from build123d import *

# Parameters (mm, degrees)
SKETCH1_W           = 2
SKETCH1_H           = 2
SKETCH1_W_2         = 1.6
SKETCH1_H_2         = 1.6
BOSS_EXTRUDE1_DEPTH = 109
SKETCH2_W           = 2
SKETCH2_H           = 2
SKETCH2_W_2         = 1.6
SKETCH2_H_2         = 1.6
BOSS_EXTRUDE2_DEPTH = 34
SKETCH3_W           = 2
SKETCH3_H           = 2
SKETCH3_W_2         = 1.6
SKETCH3_H_2         = 1.6
BOSS_EXTRUDE3_DEPTH = 6
SKETCH7_W           = 2
SKETCH7_H           = 2
SKETCH7_W_2         = 1.54
SKETCH7_H_2         = 1.54
BOSS_EXTRUDE4_DEPTH = 36
BOSS_EXTRUDE5_REACH = 28
SKETCH8_W           = 2
SKETCH8_H           = 2
SKETCH8_W_2         = 1.6
SKETCH8_H_2         = 1.6
SCALE2_SCALE        = 10
BOSS_EXTRUDE6_REACH = 1412
SKETCH9_W           = 20
SKETCH9_H           = 20
SKETCH9_W_2         = 16
SKETCH9_H_2         = 16


with BuildPart() as part:
    # Sketch1 → Boss-Extrude1 (new body)
    with BuildSketch(Plane(origin=(0, 0, 0), x_dir=(1, 0, 0), z_dir=(0, 1, 0))):
        Rectangle(SKETCH1_W, SKETCH1_H)
        Rectangle(SKETCH1_W_2, SKETCH1_H_2, mode=Mode.SUBTRACT)
    boss_extrude1 = extrude(amount=BOSS_EXTRUDE1_DEPTH)

    # Sketch2 → Boss-Extrude2 (add)
    with BuildSketch(Plane.XY.offset(1)):
        with Locations((0, 108)):
            Rectangle(SKETCH2_W, SKETCH2_H)
        with Locations((0, 108)):
            Rectangle(SKETCH2_W_2, SKETCH2_H_2, mode=Mode.SUBTRACT)
    extrude(amount=BOSS_EXTRUDE2_DEPTH)

    # Mirror1: Boss-Extrude1 across plane
    add(boss_extrude1.mirror(Plane.XY.offset(17)))

    # Sketch3 → Boss-Extrude3 (add)
    with BuildSketch(Plane.XY.offset(1)):
        with Locations((0, 1)):
            Rectangle(SKETCH3_W, SKETCH3_H)
        with Locations((0, 1)):
            Rectangle(SKETCH3_W_2, SKETCH3_H_2, mode=Mode.SUBTRACT)
    boss_extrude3 = extrude(amount=BOSS_EXTRUDE3_DEPTH)

    # Sketch7 → Boss-Extrude4 (add)
    with BuildSketch(Plane(origin=(0, 2, 0), x_dir=(1, 0, 0), z_dir=(0, 1, 0))):
        with Locations((0, -8)):
            Rectangle(SKETCH7_W, SKETCH7_H)
        with Locations((0, -8)):
            Rectangle(SKETCH7_W_2, SKETCH7_H_2, mode=Mode.SUBTRACT)
    boss_extrude4 = extrude(amount=-BOSS_EXTRUDE4_DEPTH)

    # Mirror2: Boss-Extrude3, Boss-Extrude4 across plane
    add(boss_extrude3.mirror(Plane.XY.offset(17)))
    add(boss_extrude4.mirror(Plane.XY.offset(17)))

    # Sketch8 → Boss-Extrude5 (add, up to next)
    with BuildSketch(Plane(origin=(0, 0, 25), x_dir=(-1, 0, 0), z_dir=(0, 0, -1)), mode=Mode.PRIVATE) as boss_extrude5_sk1:
        with Locations((0, -33)):
            Rectangle(SKETCH8_W, SKETCH8_H)
        with Locations((0, -33)):
            Rectangle(SKETCH8_W_2, SKETCH8_H_2, mode=Mode.SUBTRACT)
    boss_extrude5_tool1 = extrude(boss_extrude5_sk1.sketch, amount=BOSS_EXTRUDE5_REACH, mode=Mode.PRIVATE) - part.part
    add(boss_extrude5_tool1.solids().sort_by_distance((0, -32.028284, 25))[0])


with BuildPart() as part_1:
    # Scale2: scaled about (0, 0, 0)
    add(part.part.scale(SCALE2_SCALE))

    # Sketch9 → Boss-Extrude6 (add, up to next)
    with BuildSketch(Plane.XZ.offset(-1070), mode=Mode.PRIVATE) as boss_extrude6_sk1:
        with Locations((0, 169.738105544)):
            Rectangle(SKETCH9_W, SKETCH9_H)
        with Locations((0, 169.738105544)):
            Rectangle(SKETCH9_W_2, SKETCH9_H_2, mode=Mode.SUBTRACT)
    boss_extrude6_tool1 = extrude(boss_extrude6_sk1.sketch, amount=BOSS_EXTRUDE6_REACH, mode=Mode.PRIVATE) - part_1.part
    add(boss_extrude6_tool1.solids().sort_by_distance((0, 1070, 179.455263))[0])


solid = part_1.part
The listing builds one solid part. Answer for the finished solid, in the listing's coordinates (mm). Round coordinates to 2 decimals unless told otherwise and drop trailing zeros. Write each loop counter-clockwise with the first axis right and the second up, starting at its lowest first coordinate (ties: lowest second). Pieces come first, ordered by that corner, then holes. Notation, with made-up numbers: M -8,36.5 L 8,36.5 A23 cw 8,54.5 Z; hole C -8,-25 d2. An arc over 180 degrees is marked long. Write each question's results on one line, items separated by ' | '. Start each with the question number.
Item 1: Given pin 1 Ø10 at (x, y) = (-3, -161.5) entering from -Z, flat-ended and moving along its own axis, determine where the tip first touches the part or whether it passes through.
Item 2: Find section A-A on y = 65.5. Write down the section's boundary in (x, z).
Item 3: Find section B-B on z = 120. Write down the section's boundary in (x, y), and give its area (3 significant figures).
Item 4: Straight lines are drawn through the part: probe 1 along Y at (x, z) = (6.5, 213); probe 2 along Y at (x, z) = (-7.25, 322); probe 3 along Z at (x, y) = (1.5, 482). For each, find the intervals that lie inside material, in ascending order.
Item 5: Find section C-C on y = -82. Write down the section's boundary in (x, z).
Answer block:
1) pin 1: stops at z = 70
2) outline: M -10,-10 L 10,-10 L 10,10 L -10,10 Z; M -10,159.74 L 10,159.74 L 10,179.74 L -10,179.74 Z; M -10,330 L 10,330 L 10,350 L -10,350 Z; hole M -8,-8 L 8,-8 L 8,8 L -8,8 Z; hole M -8,161.74 L 8,161.74 L 8,177.74 L -8,177.74 Z; hole M -8,332 L 8,332 L 8,348 L -8,348 Z
3) outline: M -10,-340 L 10,-340 L 10,-320 L -10,-320 Z; M -10,1070 L 10,1070 L 10,1090 L -10,1090 Z; hole M -8,-338 L 8,-338 L 8,-322 L -8,-322 Z; hole M -8,1072 L 8,1072 L 8,1088 L -8,1088 Z | area: 288 mm²
4) probe 1: y = -340 to -338, -322 to -320, 1070 to 1072, 1088 to 1090 | probe 2: y = 0 to 2, 18 to 20, 1070 to 1072, 1088 to 1090 | probe 3: z = -10 to -8, 8 to 10, 159.74 to 161.74, 177.74 to 179.74, 330 to 332, 348 to 350
5) outline: M -10,70 L 10,70 L 10,90 L -10,90 Z; M -10,159.74 L 10,159.74 L 10,179.74 L -10,179.74 Z; M -10,250 L 10,250 L 10,270 L -10,270 Z; hole M -8,161.74 L 8,161.74 L 8,177.74 L -8,177.74 Z; hole M -7.7,72.3 L 7.7,72.3 L 7.7,87.7 L -7.7,87.7 Z; hole M -7.7,252.3 L 7.7,252.3 L 7.7,267.7 L -7.7,267.7 Z
